Can you work these out from the model? Positions are in its coordinate system, mm. Give positions to 0.01 mm unless a question says otherwise; leave off trailing zeros. Order: outer loops, then holes, each group sorted by start corner. A loop starts at its lowest first (then second) coordinate and runs counter-clockwise, first axis right, second up.
Item 1: If I drill on line 1 along Y through (x, z) = (0, -8.25); line 2 along X through (y, z) = (16, -6.75); line 3 along X through (y, z) = (-33, -1), over which ranges is the centre line in solid material (lowest first)?
Item 2: I want a section at C-C, the plane z = -5. Write out the boundary of the cut face in (x, y), then the cut area to 3 significant figures.
Item 3: I want a section at D-D, the plane z = 5.75. Write out the boundary of the cut face in (x, y).
Item 4: I want a section at A-A, the plane y = 0. Write out the boundary of the cut face in (x, z).
Item 5: If we mould it in two halves opening along X, with no side actions, what happens to faces 1 (the cylindrical face through (62.237, 19.599, 0.112)), 2 (the cylindrical face through (11.652, 52.472, 8.759)), 3 (the flat face through (-28, -47, -10))? For each: +X half, -X half, draft (parallel to the pull), parting line (faces both ways), or undercut.
Item 6: I'm going to push flat-ended pins straight in: pin 1 Ø1.5 at (y, z) = (18, -2.5) entering from +X; pin 2 Ø12 at (y, z) = (11.5, 7.5) entering from -X; pin 3 Ø5 at (y, z) = (-23, -6) entering from +X. Where does each tip first touch, or does it pass through?
```python
from build123d import *

# Parameters (mm, degrees)
SKETCH_1_R      = 65.25
SKETCH_1_R_2    = 50.25
EXTRUDE_1_DEPTH = 10
FILLET_1_R      = 2


with BuildPart() as part:
    # 草图1 → 凸台-拉伸1 (new, symmetric)
    with BuildSketch(Plane.XY):
        Circle(SKETCH_1_R)
        Circle(SKETCH_1_R_2, mode=Mode.SUBTRACT)
    extrude(amount=EXTRUDE_1_DEPTH, both=True)

    # 草图2 → 切除-旋转2 (revolve, cut)
    with BuildSketch(Plane(origin=(0, 0, 0), x_dir=(1, 0, 0), z_dir=(0, 1, 0)), mode=Mode.PRIVATE) as cut_revolve_2_sk:
        with BuildLine():
            Line((53.75, 10), (53.75, 7.483314774))
            ThreePointArc((53.75, 7.483314774), (57.75, 0), (53.75, -7.483314774))
            Line((53.75, -7.483314774), (53.75, -10))
            Line((53.75, -10), (42.293700596, -10))
            Line((42.293700596, -10), (42.293700596, 10))
            Line((42.293700596, 10), (53.75, 10))
        make_face()
    revolve(cut_revolve_2_sk.sketch.rotate(Axis((0, 0, -25.196328101), (0, 0, 1)), 180), axis=Axis((0, 0, -25.196328101), (0, 0, 1)), mode=Mode.SUBTRACT)

    # 圆角1
    fillet_1_edges = [part.edges().sort_by_distance(p)[0] for p in [
        (-65.25, 0, -10),
        (-65.25, 0, 10),
    ]]
    fillet(fillet_1_edges, radius=FILLET_1_R)


solid = part.part
```
Results list:
1. line 1: y = -65.23 to -53.75, 53.75 to 65.23
1. line 2: x = -63.26 to -52.31, 52.31 to 63.26
1. line 3: x = -56.29 to -47.32, 47.32 to 56.29
2. outline: circle Ø130.5 at (0, 0); hole circle Ø112.47 at (0, 0)
2. area: 3,440 mm2
3. outline: circle Ø130.5 at (0, 0); hole circle Ø111.35 at (0, 0)
4. outline: (-65.25, -8) arc R2 ccw to (-63.25, -10) - (-53.75, -10) - (-53.75, -7.48) arc R9 cw to (-53.75, 7.48) - (-53.75, 10) - (-63.25, 10) arc R2 ccw to (-65.25, 8) - close; (53.75, -10) - (63.25, -10) arc R2 ccw to (65.25, -8) - (65.25, 8) arc R2 ccw to (63.25, 10) - (53.75, 10) - (53.75, 7.48) arc R9 cw to (53.75, -7.48) - close
5. face 1: parting line
5. face 2: undercut
5. face 3: draft
6. pin 1: stops at x = 62.93
6. pin 2: stops at x = -65.02
6. pin 3: stops at x = 61.95
